```python
from build123d import *

# Parameters (mm, degrees)
SKETCH1_W           = 500
SKETCH1_H           = 350
BOSS_EXTRUDE1_DEPTH = 200
CHAMFER3_SIZE       = 100
SHELL2_T            = -5
SKETCH3_W           = 100
SKETCH3_H           = 100
BOSS_EXTRUDE3_DEPTH = 200


with BuildPart() as part:
    # Sketch1 → Boss-Extrude1 (new body)
    with BuildSketch(Plane.XY):
        with Locations((250, 175)):
            Rectangle(SKETCH1_W, SKETCH1_H)
    extrude(amount=BOSS_EXTRUDE1_DEPTH)

    # Chamfer3
    chamfer3_edges = [part.edges().sort_by_distance(p)[0] for p in [
        (250, 350, 0),
        (250, 350, 200),
        (250, 0, 0),
        (250, 0, 200),
    ]]
    chamfer(chamfer3_edges, length=CHAMFER3_SIZE - 0.0001)  # a hair under: the kernel refuses the full size

    # Shell2
    shell2_openings = [part.faces().sort_by_distance(p)[0] for p in [
        (250, 175, 0),
    ]]
    offset(amount=SHELL2_T, openings=shell2_openings, kind=Kind.INTERSECTION)

    # Sketch3 → Boss-Extrude3 (add)
    with BuildSketch(Plane.XY.offset(200)):
        with Locations((250, 175)):
            Rectangle(SKETCH3_W, SKETCH3_H)
    extrude(amount=BOSS_EXTRUDE3_DEPTH)


solid = part.part
```
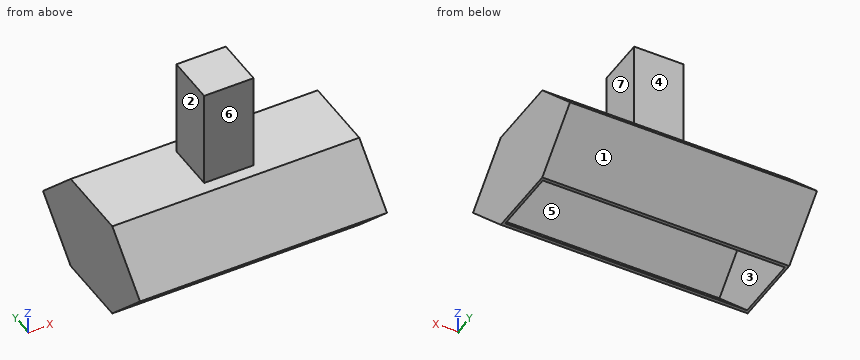
Geometry: final body of the model. Coordinates: model frame, mm. Face numbers are marked on the shaded views. A direction names the side the tool comes from. Coordinates: 2 decimals unless noted, no trailing zeros. Order: outer loops, then holes, each group sorted by start corner. A loop starts at its lowest first (then second) coordinate and runs counter-clockwise, first axis right, second up. Notation, with made-up numbers: (18.5, 9.5) -> (57.5, 9.5) arc R18 cw to (57.5, 18.5) -> close; hole circle Ø9 at (78, 1). An arc over 180 degrees is marked (long way). Use CSV: the item, a comma, the result in double quotes.
1) Section D-D on y = 237. Output: boundary loops of the cut face in (x, z).
Findings:
outline,"(0, 0) -> (5, 0) -> (5, 195) -> (495, 195) -> (495, 0) -> (500, 0) -> (500, 200) -> (0, 200) -> close"
2) Line query: line 1 (X direction, y = 213, z = 127); line 2 (Z direction, x = 479.5, y = 134); line 3 (X direction, y = 222, z = 291). Output: solid intervals per line, ascending.
Findings:
line 1,"x = 0 to 5, 495 to 500"
line 2,"z = 195 to 200"
line 3,"x = 200 to 300"
3) Access query for the marked faces 4, 5, 6 and 7. Directions: +Z, -Z, +X, -X, +Y, -Y. A direction counts if a zero-diameter tool reaches every point of the face in a straight line with its end or side. Return the directions, or none.
Findings:
face 4,"+Z, +X, -X, +Y"
face 5,"none"
face 6,"+Z, +X, -X, -Y"
face 7,"+Z, +X, +Y, -Y"
4) Pin query (flat end, axial travel): pin 1 Ø1 at (x, z) = (291.5, 247.5) entering from -Y; pin 2 Ø1.5 at (x, y) = (233, 259) entering from +Z; pin 3 Ø1 at (x, y) = (307.5, 147.5) entering from +Z. Return the tip coordinate at first contact, or that it passes through.
Findings:
pin 1,"stops at y = 125"
pin 2,"stops at z = 191.75"
pin 3,"stops at z = 200"
5) Section B-B on y = 42.5. Output: boundary loops of the cut face in (x, z).
Findings:
outline,"(0, 57.5) -> (500, 57.5) -> (500, 142.5) -> (0, 142.5) -> close; hole (5, 64.57) -> (495, 64.57) -> (495, 135.43) -> (5, 135.43) -> close"
6) Mould query, pull axis Z, two halves, no side actions, for the marked faces 1, 2 and 3. Classes: +Z half, -Z half, draft (parallel to the pull), parting line (faces both ways), or undercut.
Findings:
face 1,"-Z half"
face 2,"draft"
face 3,"undercut"
7) Section C-C on z = 54. Output: boundary loops of the cut face in (x, y).
Findings:
outline,"(0, 46) -> (500, 46) -> (500, 304) -> (0, 304) -> close; hole (5, 53.07) -> (495, 53.07) -> (495, 296.93) -> (5, 296.93) -> close"
